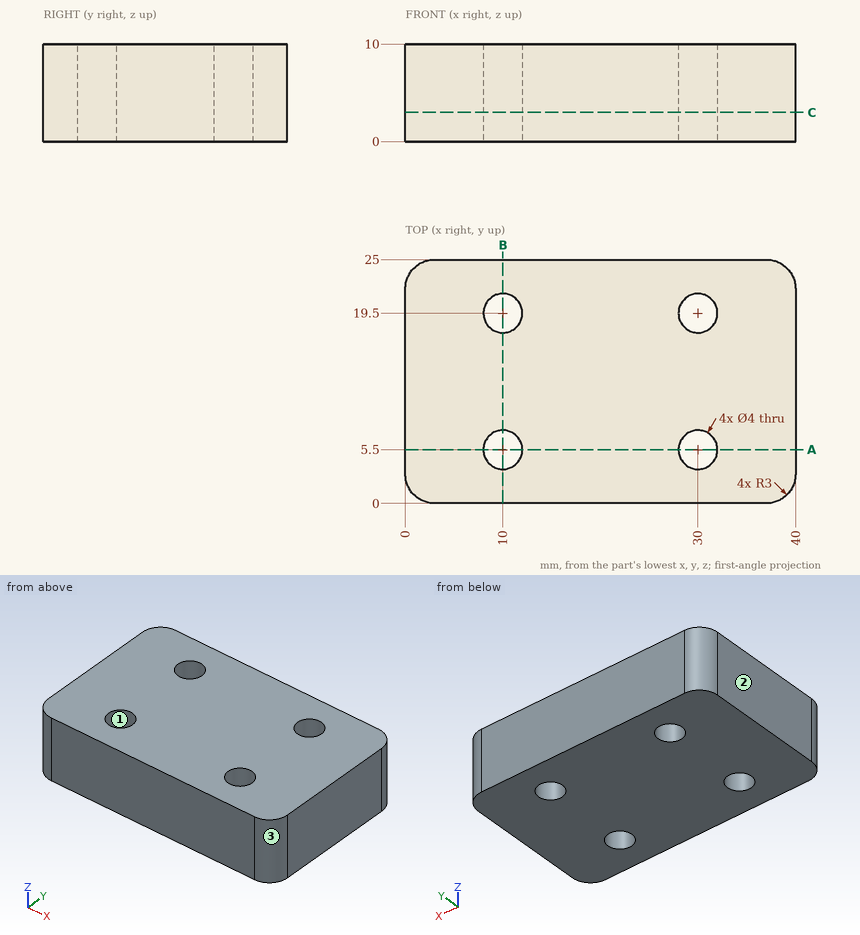
Geometry: see drawing. Coordinates: mm, zero at the bounding-box minimum. Coordinates: 2 decimals unless noted, no trailing zeros. Write each loop counter-clockwise with the first axis right and the second up, starting at its lowest first coordinate (ties: lowest second). Pieces come first, ordered by that corner, then holes. Notation, with made-up numbers: M 9,2.5 L 64,2.5 A22 ccw 64,16.5 Z; hole C -17,47 d4. An arc over 180 degrees is marked long. Use CSV: the item, a comma, the result in double quotes. Start each with the question number.
1. Cut plane B-B on x = 10. Return the cut outline in (y, z), plus the area to 3 significant figures.
2. Mould query, pull axis Y, two halves, no side actions, for the marked faces 1, 2 and 3. Classes: pulls with the +Y half, pulls with the -Y half, needs draft (parallel to the pull), parting line crosses it, or undercut.
3. Ray query, probe 1 along Y at (x, z) = (10, 3.25); probe 2 along Y at (x, z) = (31.5, 6); probe 3 along X at (y, z) = (20.5, 8.5). Return the intervals inside material, ascending.
4. Cut plane A-A on y = 5.5. Return the cut outline in (x, z), plus the area to 3 significant figures.
5. First-contact query: P1, Ø6, axis at y = 2.5, z = 7.5, coming from the -X side. Flat tip, straight axial feed; report the tip coordinate or a pass-through.
6. Cut plane C-C on z = 3. Return the cut outline in (x, y), plus the area to 3 significant figures.
Entries:
1,outline,"M 0,0 L 3.5,0 L 3.5,10 L 0,10 Z; M 7.5,0 L 17.5,0 L 17.5,10 L 7.5,10 Z; M 21.5,0 L 25,0 L 25,10 L 21.5,10 Z"
1,area,"170 mm²"
2,face 1,"undercut"
2,face 2,"needs draft"
2,face 3,"pulls with the -Y half"
3,probe 1,"0 to 3.5, 7.5 to 17.5, 21.5 to 25"
3,probe 2,"0 to 4.18, 6.82 to 18.18, 20.82 to 25"
3,probe 3,"0 to 8.27, 11.73 to 28.27, 31.73 to 40"
4,outline,"M 0,0 L 8,0 L 8,10 L 0,10 Z; M 12,0 L 28,0 L 28,10 L 12,10 Z; M 32,0 L 40,0 L 40,10 L 32,10 Z"
4,area,"320 mm²"
5,P1,"x = 0"
6,outline,"M 0,3 A3 ccw 3,0 L 37,0 A3 ccw 40,3 L 40,22 A3 ccw 37,25 L 3,25 A3 ccw 0,22 Z; hole C 10,5.5 d4; hole C 10,19.5 d4; hole C 30,5.5 d4; hole C 30,19.5 d4"
6,area,"942 mm²"
